from build123d import *

# Parameters (mm, degrees)
SKETCH2_R           = 1.95
BOSS_EXTRUDE1_DEPTH = 9
CUT_EXTRUDE1_DEPTH  = 4.4
SKETCH5_R           = 4
BOSS_EXTRUDE2_DEPTH = 0.7
CUT_EXTRUDE2_DEPTH  = 6.4


with BuildPart() as part:
    # Sketch2 → Boss-Extrude1 (new body, symmetric)
    with BuildSketch(Plane.XY):
        Circle(SKETCH2_R)
    extrude(amount=BOSS_EXTRUDE1_DEPTH, both=True)

    # Sketch4 → Cut-Extrude1 (cut)
    with BuildSketch(Plane(origin=(0, 0, -9), x_dir=(-1, 0, 0), z_dir=(0, 0, -1))):
        with BuildLine():
            Line((1, 1.674066904), (1, -1.674066904))
            ThreePointArc((1, -1.674066904), (1.95, 0), (1, 1.674066904))
        make_face()
    extrude(amount=-CUT_EXTRUDE1_DEPTH, mode=Mode.SUBTRACT)

    # Sketch5 → Boss-Extrude2 (add)
    with BuildSketch(Plane(origin=(0, 0, -9), x_dir=(-1, 0, 0), z_dir=(0, 0, -1))):
        Circle(SKETCH5_R)
    extrude(amount=BOSS_EXTRUDE2_DEPTH)

    # Sketch9 → Cut-Extrude2 (cut)
    with BuildSketch(Plane.XY.offset(9)):
        with BuildLine():
            Line((-1, 1.674066904), (-1, -1.674066904))
            ThreePointArc((-1, -1.674066904), (-1.95, 0), (-1, 1.674066904))
        make_face()
    extrude(amount=-CUT_EXTRUDE2_DEPTH, mode=Mode.SUBTRACT)


solid = part.part
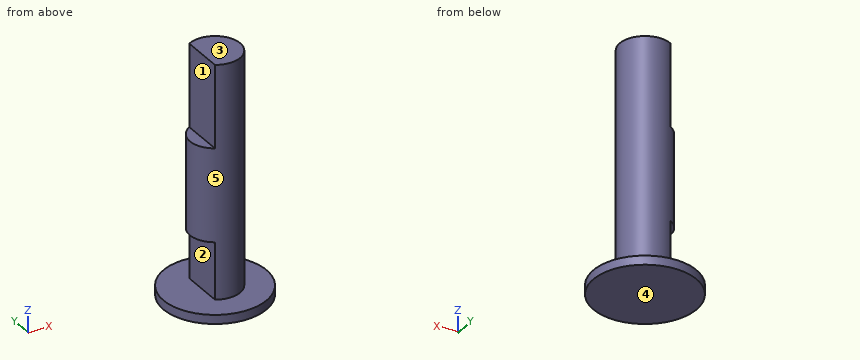
Can you work these out from the model? Positions are in its coordinate system, mm. Face numbers are marked on the shaded views. A direction names the side the tool comes from. Give positions to 0.01 mm unless a question says otherwise; leave off trailing zeros. Write each loop counter-clockwise with the first axis right and the second up, starting at its lowest first coordinate (ties: lowest second). Pieces come first, ordered by that corner, then holes. Notation, with made-up numbers: (-39.5, 86.25) -> (-23.5, 86.25) arc R31 ccw to (-23.5, 112.25) -> close; hole circle Ø10 at (29.5, 25.5). An arc over 180 degrees is marked (long way). Answer as a JSON object with one key per item and string values. Group by question number.
Item 1: Suppose I cut it at D-D (z = 1). Please give me the cut outline in (x, y), plus the area to 3 significant figures.
Item 2: I'm going to push flat-ended pins straight in: P1, Ø1.7, axis at y = -0.5, z = 5.5, coming from the -X side; P2, Ø4, axis at y = 2, z = -6, coming from the -X side; P3, Ø4, axis at x = 0, z = 4, coming from the -Y side. Where does each tip first touch, or does it pass through?
Item 3: Suppose I cut it at C-C (z = -8). Please give me the cut outline in (x, y), plus the area to 3 significant figures.
Item 4: Please list where these lines run through material, in increasing order: line 1 (Z direction, x = -2, y = -1.5); line 2 (Y direction, x = 1, z = 4.75); line 3 (Y direction, x = -0.75, z = -7). Write a range as [from, to].
Item 5: Suppose I cut it at A-A (y = 0). Please give me the cut outline in (x, z).
Item 6: Suppose I cut it at B-B (x = 0). Please give me the cut outline in (y, z), plus the area to 3 significant figures.
Item 7: For the marked faces 1, 2, 3, 4 and 5, which set-ups out of +Z, -Z, +X, -X, +Y, -Y let a thin tool reach every point of the face, with its end or its side?
Findings:
{
 "1": {"outline": "circle Ø3.9 at (0, 0)", "area": "11.9 mm²"},
 "2": {"P1": "stops at x = -1", "P2": "stops at x = -1.86", "P3": "stops at y = -1.95"},
 "3": {"outline": "(-1, -1.67) arc R1.95 ccw (long way) to (-1, 1.67) -> close", "area": "9.69 mm²"},
 "4": {"line 1": "z = [-9.7, -9]", "line 2": "y = [-1.67, 1.67]", "line 3": "y = [-1.8, 1.8]"},
 "5": {"outline": "(-4, -9.7) -> (4, -9.7) -> (4, -9) -> (1.95, -9) -> (1.95, 9) -> (-1, 9) -> (-1, 2.6) -> (-1.95, 2.6) -> (-1.95, -4.6) -> (-1, -4.6) -> (-1, -9) -> (-4, -9) -> close"},
 "6": {"outline": "(-4, -9.7) -> (4, -9.7) -> (4, -9) -> (1.95, -9) -> (1.95, 9) -> (-1.95, 9) -> (-1.95, -9) -> (-4, -9) -> close", "area": "75.8 mm²"},
 "7": {"face 1": "+Z, -X, +Y, -Y", "face 2": "-X, +Y, -Y", "face 3": "+Z, +X, -X, +Y, -Y", "face 4": "-Z, +X, -X, +Y, -Y", "face 5": "+Z"}
}
